Read the model definition and answer for the solid it produces. Units are mm, in the model's axes. A direction names the side the tool comes from. Coordinates: 2 decimals unless noted, no trailing zeros. Loops run counter-clockwise (first coordinate to the right, second up) from the corner with the lowest first, then second, coordinate; pieces in that order, holes last. Notation, with made-up numbers: (45, -19) - (71, -19) arc R33 ccw to (71, 14) - close; hole circle Ø11 at (8, -22.5). An arc over 180 degrees is marked (long way). Use one line per item in the form item = value. Start each with the question number.
1) A cutting plane is placed at A-A (x = -107). Give the vertices of the cut face in (y, z).
2) A cutting plane is placed at C-C (y = 57.5). State how many separate pieces and enclosed holes the cut face has, and give its area (3 significant figures).
3) Which of the six approach directions +Z, -Z, +X, -X, +Y, -Y give full straight-line access (tool end or side, diameter ignored) to faces 3 (the face through (-50.8, 51.6, 3)), 4 (the face through (-83, 89, 3))?
4) Each of these flat-tipped pins is pushed along its axis until it touches: P1, Ø1.8, axis at y = 89, z = 2, coming from the +X side; P2, Ø3, axis at x = -24.6, y = 72.2, coming from the -Z side; P3, Ø3, axis at x = -49.5, z = 4.5, coming from the +Y side; P4, Ø1.5, axis at x = -80, z = 0.5, coming from the -Y side. Where does it stop, or does it pass through?
5) Consider line 1 (Y direction, x = -24.6, z = 4.4); line 2 (Y direction, x = -31.3, z = 3.45); line 3 (X direction, y = 82, z = 5.6). Determine where each line is inside the solid, lowest interval first.
6) The mould has two halves that part along X. Classify faces 1 (the face through (-63.3, 48.4, 3)), 2 (the face through (-79, 51, 6)): released by +X, released by -X, zero draft, split by the parting line, or undercut.
7) A cutting plane is placed at B-B (x = -39.3). Give the vertices of the cut face in (y, z).
Autodesk Fusion 360 part; units mm, degrees
sketch "Esquisse1" plane through (0, 0, 0) normal (0, 0, 1) x (1, 0, 0)
  line L0 (0, 0) -> (-127.5, 0)
  line L1 (-127.5, 0) -> (-127.5, 100)
  line L2 (-127.5, 100) -> (0, 100)
  line L3 (0, 100) -> (0, 0)
  ellipse E0 centre (-10, 50) end of major axis (0, 50) minor radius 50
  line L4 (-20, 50) -> (0, 50)
  line L5 (-10, 0) -> (-10, 100)
  ellipse E1 centre (-125, 50) end of major axis (-127.5, 50) minor radius 50
  line L6 (-122.5, 50) -> (-127.5, 50)
  line L7 (-125, 100) -> (-125, 0)
  line L8 (-10, 100) -> (-83, 100)
  line L9 (-83, 100) -> (-83, 77)
  line L10 (-83, 77) -> (-10, 77)
  line L11 (-10, 77) -> (-10, 100)
  line L12 (-10, 0) -> (-83, 0)
  line L13 (-83, 0) -> (-83, 23)
  line L14 (-83, 23) -> (-10, 23)
  line L15 (-10, 23) -> (-10, 0)
  dimension "d1" = 127.5
  dimension "d2" = 73
  dimension "d3" = 23
  dimension "d4" = 73
  dimension "d5" = 23
extrude "Extrusion1" add sketch "Esquisse1" along normal blind 6 contours E0 L4 L5 L15 | E0 L4 L5 L11 | L0 L2 E0 E1 L9 L10 L13 L14 | E0 L4 L5 L14 | E0 L4 L5 L10 | E1 L6 L7 | E1 L6 L7 | E1 L6 L7 | E1 L6 L7
sketch "Esquisse2" plane through (0, 0, 6) normal (0, 0, 1) x (-1, 0, 0)
  line L0 (83, 0) -> (83, -23)
  line L1 (83, -23) -> (10, -23)
  line L2 (10, -23) -> (10, 0)
  ellipse E0 centre (10, -50) end of major axis (10, -100) minor radius 10 (10, 0) -> (10, -100) ccw
  line L3 (10, -100) -> (10, -77)
  line L4 (10, -77) -> (83, -77)
  line L5 (83, -77) -> (83, -100)
  line L6 (83, -100) -> (125, -100)
  ellipse E1 centre (125, -50) end of major axis (125, 0) minor radius 2.5 (125, -100) -> (125, 0) ccw
  line L7 (125, 0) -> (83, 0)
  circle A0 centre (107, -50) radius 10
  circle A1 centre (119.6, -16) radius 3
  circle A2 centre (119.6, -84) radius 3
  line L8 (0, -100) -> (0, 0)
  line L9 (127.5, -100) -> (0, -100)
  circle A3 centre (6, -30.25) radius 3
  line L10 (10, 0) -> (83, 0)
  circle A4 centre (6, -69.75) radius 3
  dimension "d8" = 20
  dimension "d9" = 6
  dimension "d10" = 16
  dimension "d11" = 119.6
  dimension "d12" = 6
  dimension "d13" = 119.6
  dimension "d14" = 16
  dimension "d15" = 6
  dimension "d16" = 30.25
  dimension "d17" = 6
  dimension "d18" = 6
  dimension "d19" = 6
  dimension "d20" = 30.25
  dimension "d49" = 107
extrude "Extrusion2" cut sketch "Esquisse2" against normal blind 7 contours A0 | A1 | A2 | A3 | A4
sketch "Esquisse3" plane through (0, 0, 6) normal (0, 0, 1) x (-1, 0, 0)
  circle A0 centre (119.6, -16) radius 3
  circle A1 centre (107, -50) radius 10
  circle A2 centre (6, -30.25) radius 3
  circle A3 centre (119.6, -84) radius 3
  circle A4 centre (6, -69.75) radius 3
  line L0 (83, 0) -> (83, -23)
  line L1 (83, -23) -> (10, -23)
  line L2 (10, -23) -> (10, 0)
  ellipse E0 centre (10, -50) end of major axis (10, -100) minor radius 10 (10, 0) -> (10, -100) ccw
  line L3 (10, -100) -> (10, -77)
  line L4 (10, -77) -> (83, -77)
  line L5 (83, -77) -> (83, -100)
  line L6 (83, -100) -> (125, -100)
  ellipse E1 centre (125, -50) end of major axis (125, 0) minor radius 2.5 (125, -100) -> (125, 0) ccw
  line L7 (125, 0) -> (83, 0)
  circle A5 centre (39.3, -49.9) radius 1.5
  line L8 (0, -100) -> (0, 0)
  line L9 (10, 0) -> (83, 0)
  circle A6 centre (50.8, -49.9) radius 1.5
  circle A7 centre (63.3, -49.9) radius 1.5
  line L10 (0, 0) -> (127.5, 0)
  circle A8 centre (31.3, -26.5) radius 1.5
  circle A9 centre (31.3, -42.5) radius 1.5
  circle A10 centre (101.15, -18) radius 1.5
  circle A11 centre (112.9372, -39) radius 1.5
  circle A12 centre (94.5, -50) radius 1.5
  circle A13 centre (118.55, -8.8) radius 1.5
  circle A14 centre (120.65, -23.2) radius 1.5
  circle A15 centre (24.6, -27.8) radius 1.25
  circle A16 centre (7, -23) radius 1.5
  circle A17 centre (5.5, -37.5) radius 1.5
  point P0 (107, -50)
  dimension "d23" = 3
  dimension "d24" = 39.3
  dimension "d25" = 49.9
  dimension "d26" = 3
  dimension "d27" = 49.9
  dimension "d28" = 50.8
  dimension "d29" = 3
  dimension "d30" = 63.3
  dimension "d31" = 49.9
  dimension "d32" = 3
  dimension "d33" = 26.5
  dimension "d34" = 31.3
  dimension "d35" = 3
  dimension "d36" = 31.3
  dimension "d37" = 42.5
  dimension "d38" = 3
  dimension "d39" = 18
  dimension "d40" = 101.15
  dimension "d41" = 3
  dimension "d44" = 3
  dimension "d45" = 50
  dimension "d46" = 94.5
  dimension "d51" = 12.5
  dimension "d52" = 39
  dimension "d53" = 3
  dimension "d54" = 8.8
  dimension "d55" = 118.55
  dimension "d56" = 3
  dimension "d57" = 120.65
  dimension "d58" = 23.2
  dimension "d59" = 2.5
  dimension "d60" = 27.8
  dimension "d61" = 24.6
  dimension "d62" = 3
  dimension "d63" = 23
  dimension "d64" = 7
  dimension "d65" = 3
  dimension "d66" = 5.5
  dimension "d67" = 37.5
extrude "Extrusion3" cut sketch "Esquisse3" against normal blind 6 contours A5 | A6 | A7 | A8 | A9 | A10 | A11 | A12 | A13 | A14 | A15 | A16 | A17
ref_plane "Plan de construction1" through (-104, 50, 3) normal (0, 1, 0) x (-1, 0, 0)
mirror "Symétrie miroir1" about plane through (-104, 50, 3) normal (0, 1, 0) of "Extrusion3"
Found:
q1.outline = (0, 0) - (40, 0) - (40, 6) - (0, 6) - close; (60, 0) - (100, 0) - (100, 6) - (60, 6) - close
q2.separate_pieces = 3
q2.enclosed_holes = 0
q2.area = 667 mm^2
q3.face_3 = +Z, -Z
q3.face_4 = +Z, -Z, +Y
q4.P1 = -3.52
q4.P2 = 0
q4.P3 = 77
q4.P4 = 23
q5.line_1 = 23 to 26.55, 29.05 to 70.95, 73.45 to 77
q5.line_2 = 23 to 25, 28 to 41, 44 to 56, 59 to 72, 75 to 77
q5.line_3 = -126.92 to -121.84, -117.36 to -102.65, -99.65 to -83, -10 to -2.32
q6.face_1 = undercut
q6.face_2 = zero draft
q7.outline = (23, 0) - (48.4, 0) - (48.4, 6) - (23, 6) - close; (51.6, 0) - (77, 0) - (77, 6) - (51.6, 6) - close
